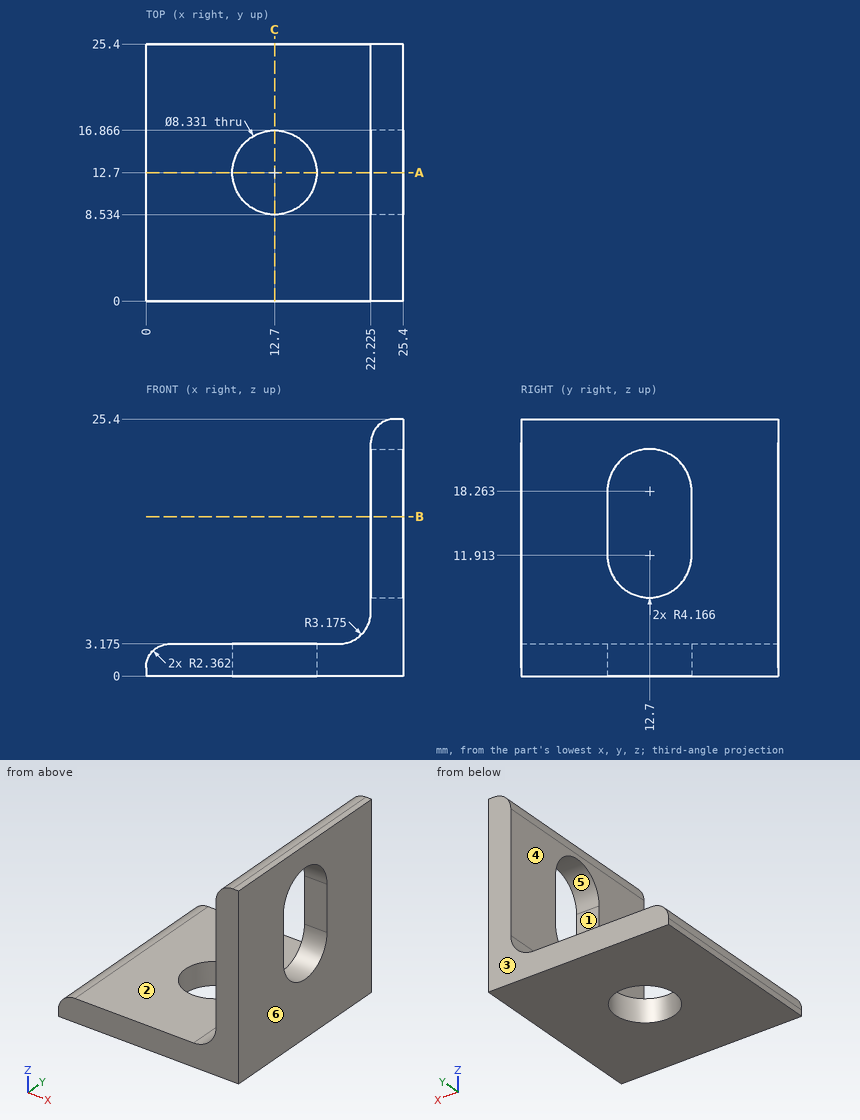
For this review, use the dimensioned drawing (mm, ordinates from the lowest corner) and the shaded views. A direction names the side the tool comes from. Give positions to 0.01 mm unless a question says otherwise; leave off trailing zeros. Order: outer loops, then holes, each group sorted by start corner. A loop starts at its lowest first (then second) coordinate and runs counter-clockwise, first axis right, second up.
1) Take a section at B-B (z = 15.75). Give the boundary of the cut face in (x, y) (1 decimal).
2) The part is to be moulded in two halves that separate along Y. For the marked faces 1, 2 and 3, say which applies: released by +Y, released by -Y, zero draft, split by the parting line, or undercut.
3) For the marked faces 4, 5 and 6, list the 3-axis set-ups (+Z, -Z, +X, -X, +Y, -Y) from which the entire face can be reached by the end or side of a thin tool; tool diameter is ignored.
4) Wall thickness on line 1 (Y direction, x = 12.7, z = 1.4) (1 decimal); line 2 (Z direction, x = 17.75, y = 1.75) (1 decimal); line 3 (Z direction, x = 23.5, y = 16.5) (1 decimal): over which ranges is each line inside the solid? List them lowest first.
5) Insertion check: pin 1 (13.5 mm diameter, centred on x = 14, y = 13, fed in from +Z); pin 2 (5 mm diameter, centred on y = 18.5, z = 15.5, fed in from -X) (3 decimals); pin 3 (3.5 mm diameter, centred on x = 23, z = 15.5, fed in from -Y); pin 4 (1.5 mm diameter, centred on y = 10, z = 15, fed in from -X). Each pin has a flat end and moves straight along its axis. Give the tip position at first contact, or say it passes through.
6) Take a section at C-C (x = 12.7). Give the boundary of the cut face in (y, z) (1 decimal).
7) Take a section at A-A (y = 12.7). State how many separate pieces and enclosed holes the cut face has.
Derived:
1. outline: (22.2, 0) - (25.4, 0) - (25.4, 8.5) - (22.2, 8.5) - close; (22.2, 16.9) - (25.4, 16.9) - (25.4, 25.4) - (22.2, 25.4) - close
2. face 1: undercut
2. face 2: zero draft
2. face 3: released by +Y
3. face 4: +Z, -X, +Y, -Y
3. face 5: +X, -X
3. face 6: +Z, -Z, +X, +Y, -Y
4. line 1: y = 0 to 8.5, 16.9 to 25.4
4. line 2: z = 0 to 3.2
4. line 3: z = 0 to 10.2, 20 to 25.1
5. pin 1: stops at z = 3.67
5. pin 2: stops at x = 22.225
5. pin 3: stops at y = 0
5. pin 4: passes through
6. outline: (0, 0) - (8.5, 0) - (8.5, 3.2) - (0, 3.2) - close; (16.9, 0) - (25.4, 0) - (25.4, 3.2) - (16.9, 3.2) - close
7. separate pieces: 3
7. enclosed holes: 0
